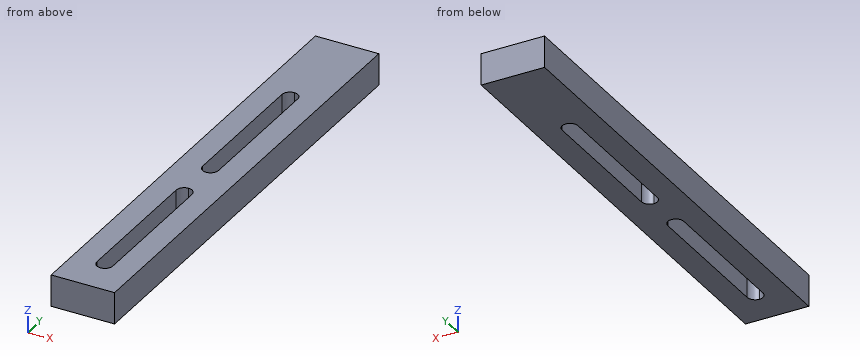
from build123d import *

# Parameters (mm, degrees)
F0_W     = 20
F0_H     = 150
F1_DEPTH = 10
F2_W     = 5
F2_H     = 50
F3_DEPTH = 25
F4_R     = 2.49999


# Not quite as in the source:
# - a fillet or chamfer is up to 0.001 mm smaller than in the source, because OpenCascade refuses the exact size


with BuildPart() as f1:
    # F0 (on Top) → F1 (new body)
    with BuildSketch(Plane.XY):
        with Locations((10, 75)):
            Rectangle(F0_W, F0_H)
    extrude(amount=F1_DEPTH)

    # F2 (on face) → F3 (cut)
    with BuildSketch(Plane.XY.offset(10)):
        with Locations((10, 95)):
            Rectangle(F2_W, F2_H)
        with Locations((10, 35)):
            Rectangle(F2_W, F2_H)
    extrude(amount=-F3_DEPTH, mode=Mode.SUBTRACT)

    # F4 (radius 2.5 in the source; OpenCascade refuses exactly that, so slightly less here)
    f4_edges = [f1.edges().sort_by_distance(p)[0] for p in [
        (12.5, 60, 5),
        (7.5, 60, 5),
        (7.5, 120, 5),
        (12.5, 120, 5),
        (7.5, 70, 5),
        (7.5, 10, 5),
        (12.5, 10, 5),
        (12.5, 70, 5),
    ]]
    fillet(f4_edges, radius=F4_R)


solid = f1.part
Model file for the job. Use its own axes, mm. Coordinates: 2 decimals unless noted, no trailing zeros. Loops run counter-clockwise (first coordinate to the right, second up) from the corner with the lowest first, then second, coordinate; pieces in that order, holes last. Notation, with made-up numbers: (89, 73.25) -> (105, 73.25) arc R18 ccw to (105, 82.25) -> close; hole circle Ø8 at (16.25, 16). An arc over 180 degrees is marked (long way). Use one line per item in the form item = value. Start each with the question number.
(1) Cut at A-A on z = 3. Give the number of separate pieces and of enclosed holes in the cut face, and give its area (3 significant figures).
(2) Flat gauge pin, fed straight in: pin 1 (5 mm diameter, centred on x = 17, z = 7, fed in from -Y). Where does the tip first touch, or does it go through?
(3) Probe probe 1 along X at (y, z) = (46, 2.5); probe 2 along Y at (x, z) = (11.25, 1.25); probe 3 along Y at (x, z) = (10.75, 1.25). List the from-to ranges inside material, lowest first. Write a range as from..to.
(4) Cut at C-C on x = 11.25. Give the cut face in (y, z), and give its area (3 significant figures).
(5) Cut at B-B on y = 96. Give the cut face in (x, z), and give its area (3 significant figures).
Values:
q1.separate_pieces = 1
q1.enclosed_holes = 2
q1.area = 2,510 mm2
q2.pin_1 = 0
q3.probe_1 = 0..7.5, 12.5..20
q3.probe_2 = 0..10.33, 59.67..70.33, 119.67..150
q3.probe_3 = 0..10.12, 59.88..70.12, 119.88..150
q4.outline = (0, 0) -> (10.33, 0) -> (10.33, 10) -> (0, 10) -> close; (59.67, 0) -> (70.33, 0) -> (70.33, 10) -> (59.67, 10) -> close; (119.67, 0) -> (150, 0) -> (150, 10) -> (119.67, 10) -> close
q4.area = 513 mm2
q5.outline = (0, 0) -> (7.5, 0) -> (7.5, 10) -> (0, 10) -> close; (12.5, 0) -> (20, 0) -> (20, 10) -> (12.5, 10) -> close
q5.area = 150 mm2
